Design review of the part shown in the three views and the two pictorial views. Dimensions are in mm from the part's minimum x, y and z. A direction names the side the tool comes from. Give positions to 0.01 mm unless a question says otherwise; leave off trailing zeros. Write each loop counter-clockwise with the first axis right and the second up, starting at its lowest first coordinate (ties: lowest second). Pieces come first, ordered by that corner, then holes.
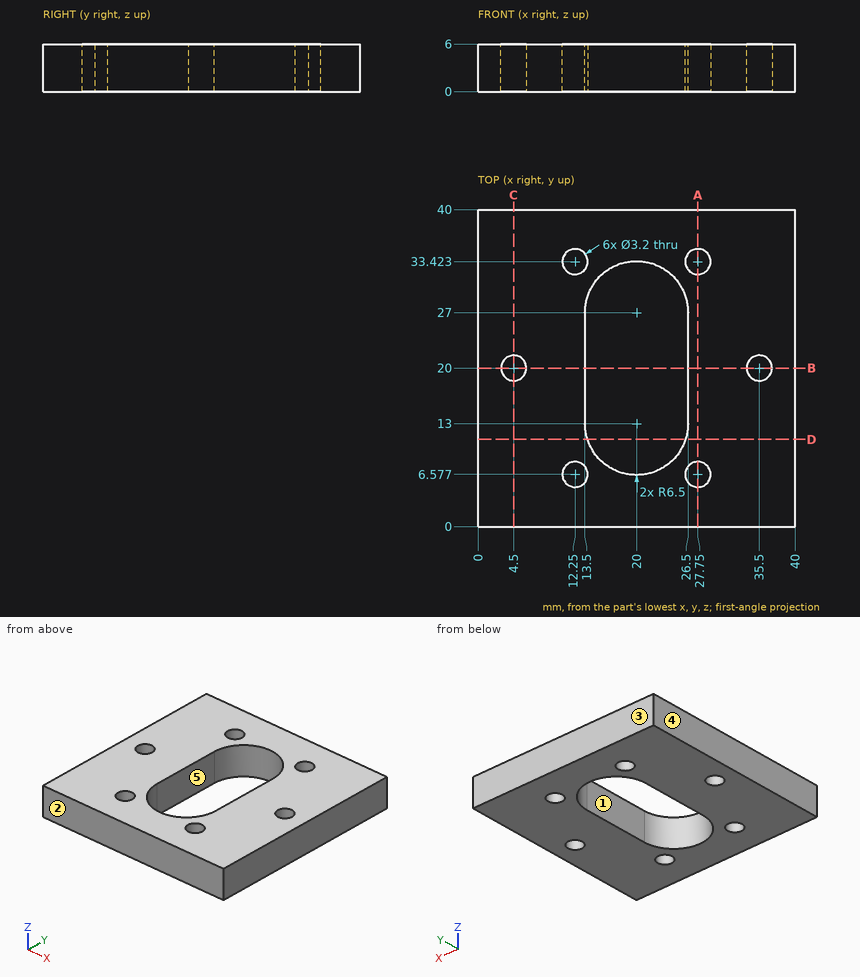
(1) Consider section A-A, the plane x = 27.75. Give the boundary of the cut face in (y, z), then the cut area to 3 significant figures.
Resolved:
outline: (0, 0) - (4.98, 0) - (4.98, 6) - (0, 6) - close; (8.18, 0) - (31.82, 0) - (31.82, 6) - (8.18, 6) - close; (35.02, 0) - (40, 0) - (40, 6) - (35.02, 6) - close
area: 202 mm2
(2) Clearance check with a flat-ended pin moving along its axis: P1, Ø1.5, axis at x = 16.5, z = 3, coming from the -Y side. State where the tip first meets the part, or that it passes through.
Resolved:
P1: stops at y = 0
(3) To check wall thickness, follow L1, parallel to Y at x = 12.25, z = 3.95; L2, parallel to X at y = 22, z = 0.65; L3, parallel to Y at x = 35.5, z = 4.55. State the ranges of each line that lie inside material, in increasing order.
Resolved:
L1: y = 0 to 4.98, 8.18 to 31.82, 35.02 to 40
L2: x = 0 to 13.5, 26.5 to 40
L3: y = 0 to 18.4, 21.6 to 40
(4) Mouldability with a two-part tool opening along Y and no side actions: class the marked faces 1, 2 and 3 as pulls with the +Y half, pulls with the -Y half, needs draft (parallel to the pull), parting line crosses it, or undercut.
Resolved:
face 1: undercut
face 2: pulls with the -Y half
face 3: pulls with the +Y half
(5) Tool access review of the marked faces 4 and 5: name each direction out of +Z, -Z, +X, -X, +Y, -Y from which nothing blocks a thin tool from reaching the whole face with its end or side.
Resolved:
face 4: +Z, -Z, -X, +Y, -Y
face 5: +Z, -Z
(6) Consider section B-B, the plane y = 20. Give the boundary of the cut face in (x, z).
Resolved:
outline: (0, 0) - (2.9, 0) - (2.9, 6) - (0, 6) - close; (6.1, 0) - (13.5, 0) - (13.5, 6) - (6.1, 6) - close; (26.5, 0) - (33.9, 0) - (33.9, 6) - (26.5, 6) - close; (37.1, 0) - (40, 0) - (40, 6) - (37.1, 6) - close
(7) Consider section C-C, the plane x = 4.5. Give the boundary of the cut face in (y, z).
Resolved:
outline: (0, 0) - (18.4, 0) - (18.4, 6) - (0, 6) - close; (21.6, 0) - (40, 0) - (40, 6) - (21.6, 6) - close
(8) Consider section D-D, the plane y = 11. Give the boundary of the cut face in (x, z) (1 decimal), then the cut area to 3 significant figures.
Resolved:
outline: (0, 0) - (13.8, 0) - (13.8, 6) - (0, 6) - close; (26.2, 0) - (40, 0) - (40, 6) - (26.2, 6) - close
area: 166 mm2
